The model under review builds one solid part; all positions refer to its coordinate system, in mm. A direction names the side the tool comes from. Coordinates: 2 decimals unless noted, no trailing zeros. Write each loop counter-clockwise with the first axis right and the second up, starting at its lowest first coordinate (ties: lowest second). Pieces come first, ordered by that corner, then holes. Notation, with made-up numbers: M 49.5,24 L 75.5,24 A26 ccw 75.5,54 Z; hole C 69,-17 d6. An arc over 180 degrees is marked long. Answer as CSV lines item,"result". Start each with the question number.
from build123d import *

# Parameters (mm, degrees)
SKETCH8_W           = 131.76
SKETCH8_H           = 95.69
SKETCH8_R           = 3.43
SKETCH8_W_2         = 73.4
SKETCH8_H_2         = 33.99
BOSS_EXTRUDE4_DEPTH = 40
SKETCH9_R           = 8
CUT_EXTRUDE2_DEPTH  = 8


with BuildPart() as part:
    # Sketch8 → Boss-Extrude4 (new body)
    with BuildSketch(Plane(origin=(0, 0, 0), x_dir=(1, 0, 0), z_dir=(0, 1, 0))):
        with Locations((-55.88, 37.845)):
            Rectangle(SKETCH8_W, SKETCH8_H)
        with Locations((-100.58, 12.85)):
            Circle(SKETCH8_R, mode=Mode.SUBTRACT)
        with Locations((-100.58, 62.84)):
            Circle(SKETCH8_R, mode=Mode.SUBTRACT)
        with Locations((-11.18, 62.84)):
            Circle(SKETCH8_R, mode=Mode.SUBTRACT)
        with Locations((-11.18, 12.85)):
            Circle(SKETCH8_R, mode=Mode.SUBTRACT)
        with Locations((-55.88, 37.845)):
            Rectangle(SKETCH8_W_2, SKETCH8_H_2, mode=Mode.SUBTRACT)
    extrude(amount=BOSS_EXTRUDE4_DEPTH)

    # Sketch9 → Cut-Extrude2 (cut)
    with BuildSketch(Plane.XZ):
        with Locations((-100.58, -12.85)):
            Circle(SKETCH9_R)
        with Locations((-11.18, -12.85)):
            Circle(SKETCH9_R)
        with Locations((-11.18, -62.84)):
            Circle(SKETCH9_R)
        with Locations((-100.58, -62.84)):
            Circle(SKETCH9_R)
    extrude(amount=-CUT_EXTRUDE2_DEPTH, mode=Mode.SUBTRACT)


solid = part.part
1) Take a section at B-B on y = 21. Give the boundary of the cut face in (x, z), and give its area (3 significant figures).
2) To check wall thickness, follow line 1 (Z direction, x = -11, y = 5); line 2 (Z direction, x = -11, y = 24); line 3 (X direction, y = 3, z = -52). State the ranges of each line that lie inside material, in increasing order. Write a range as [from, to].
3) Take a section at D-D on x = -100.58. Give the boundary of the cut face in (y, z), and give its area (3 significant figures).
4) Clearance check with flat-ended pins moving along their axes: pin 1 Ø17.5 at (x, z) = (-13, -64) entering from -Y; pin 2 Ø9 at (x, z) = (-11.18, -62.84) entering from -Y; pin 3 Ø5.5 at (x, z) = (-100.58, -62.84) entering from +Y. State where each tip first meets the part, or that it passes through.
5) Mouldability with a two-part tool opening along X and no side actions: class faces 1 (the flat face through (-57, 0, -60)), 2 (the flat face through (-121.76, 20, -37)), 3 (the cylindrical face through (-96.279, 3.944, -6.104)) as +X half, -X half, draft (parallel to the pull), parting line (faces both ways), or undercut.
6) Tool access review of faces 4 (the flat face through (-56, 20, -20.85)), 5 (the flat face through (-57, 40, -17)), 6 (the flat face through (-97, 8, -63)): name each direction out of +Z, -Z, +X, -X, +Y, -Y from which nothing blocks a thin tool from reaching the whole face with its end or side.
7) Take a section at C-C on z = -12.85. Give the boundary of the cut face in (x, y), and give its area (3 significant figures).
8) Take a section at A-A on x = -57. Give the boundary of the cut face in (y, z), and give its area (3 significant figures).
Results:
1,outline,"M -121.76,-85.69 L 10,-85.69 L 10,10 L -121.76,10 Z; hole C -100.58,-62.84 d6.86; hole C -100.58,-12.85 d6.86; hole M -92.58,-54.84 L -19.18,-54.84 L -19.18,-20.85 L -92.58,-20.85 Z; hole C -11.18,-62.84 d6.86; hole C -11.18,-12.85 d6.86"
1,area,"9,970 mm²"
2,line 1,"z = [-85.69, -70.84], [-54.84, -20.85], [-4.85, 10]"
2,line 2,"z = [-85.69, -66.27], [-59.41, -16.28], [-9.42, 10]"
2,line 3,"x = [-121.76, -92.58], [-19.18, 10]"
3,outline,"M 0,-85.69 L 40,-85.69 L 40,-66.27 L 8,-66.27 L 8,-70.84 L 0,-70.84 Z; M 0,-54.84 L 8,-54.84 L 8,-59.41 L 40,-59.41 L 40,-16.28 L 8,-16.28 L 8,-20.85 L 0,-20.85 Z; M 0,-4.85 L 8,-4.85 L 8,-9.42 L 40,-9.42 L 40,10 L 0,10 Z"
3,area,"3,130 mm²"
4,pin 1,"stops at y = 0"
4,pin 2,"stops at y = 8"
4,pin 3,"passes through"
5,face 1,"draft"
5,face 2,"-X half"
5,face 3,"undercut"
6,face 4,"+Y, -Y"
6,face 5,"+Z, -Z, +X, -X, +Y"
6,face 6,"-Y"
7,outline,"M -121.76,0 L -108.58,0 L -108.58,8 L -104.01,8 L -104.01,40 L -121.76,40 Z; M -97.15,8 L -92.58,8 L -92.58,0 L -19.18,0 L -19.18,8 L -14.61,8 L -14.61,40 L -97.15,40 Z; M -7.75,8 L -3.18,8 L -3.18,0 L 10,0 L 10,40 L -7.75,40 Z"
7,area,"4,580 mm²"
8,outline,"M 0,-85.69 L 40,-85.69 L 40,-54.84 L 0,-54.84 Z; M 0,-20.85 L 40,-20.85 L 40,10 L 0,10 Z"
8,area,"2,470 mm²"
